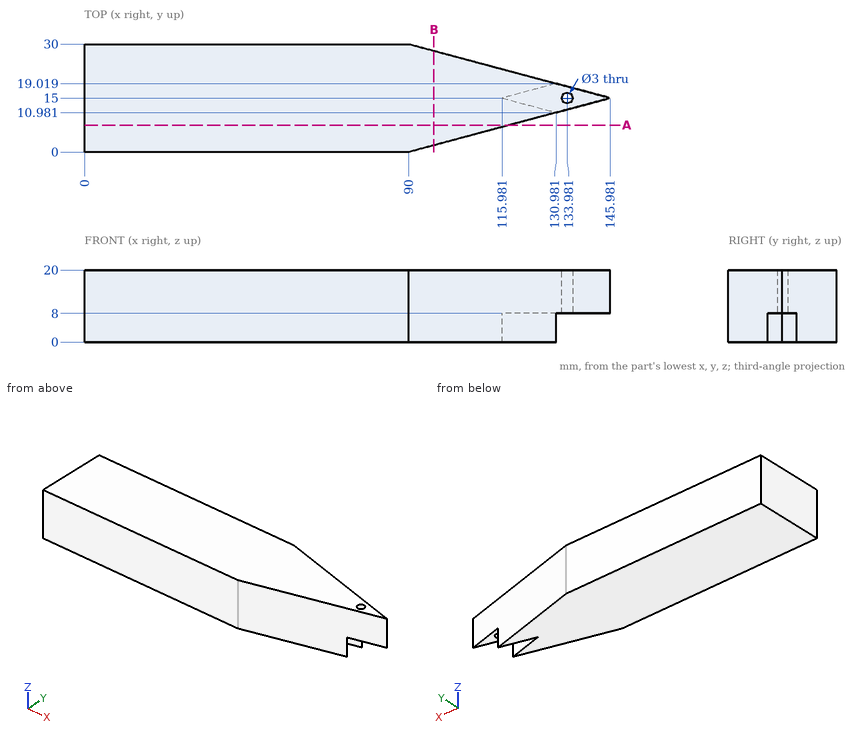
Here's the drawing with two shaded views (mm, measured from the low corner). I have some questions. Give positions to 0.01 mm unless a question says otherwise; leave off trailing zeros. Loops run counter-clockwise (first coordinate to the right, second up) from the corner with the lowest first, then second, coordinate; pieces in that order, holes last. Notation, with made-up numbers: (24.25, -21.75) -> (64.25, -21.75) arc R10 cw to (64.25, -16.75) -> close; hole circle Ø6 at (15.25, 1.25). An arc over 180 degrees is marked (long way). Answer as a JSON object with one key per item and string values. Group by question number.
Item 1: Imagine slicing it at B-B on x = 97. Write out the boundary of the cut face in (y, z).
Item 2: Imagine slicing it at A-A on y = 7.5. Write out the boundary of the cut face in (x, z), then the cut area to 3 significant figures.
Item 3: I need wall thicknesses on L1, parallel to Z at x = 137, y = 13.25; L2, parallel to Y at x = 134, z = 19; L3, parallel to Y at x = 114.5, z = 18 (1 decimal). Which ranges of each line are inside material? Lowest first, please.
Item 4: Will these pins go through, and if not, where does the flat tip stop? pin 1 (6.5 mm diameter, centred on x = 133, y = 14.5, fed in from -Z); pin 2 (1.5 mm diameter, centred on y = 22.5, z = 8.5, fed in from -X); pin 3 (1.8 mm diameter, centred on x = 133.98, y = 15, fed in from -Z); pin 4 (8 mm diameter, centred on y = 13, z = 2.5, fed in from +X).
Answer list:
{
 "1": {"outline": "(1.88, 0) -> (28.12, 0) -> (28.12, 20) -> (1.88, 20) -> close"},
 "2": {"outline": "(0, 0) -> (117.99, 0) -> (117.99, 20) -> (0, 20) -> close", "area": "2,360 mm2"},
 "3": {"L1": "z = 8 to 20", "L2": "y = 11.79 to 13.5, 16.5 to 18.21", "L3": "y = 6.6 to 23.4"},
 "4": {"pin 1": "stops at z = 8", "pin 2": "stops at x = 0", "pin 3": "passes through", "pin 4": "stops at x = 130.98"}
}
